For this review, take the finished solid that the model builds, in its own axes (mm). Face numbers are marked on the shaded views. Round coordinates to 2 decimals unless told otherwise and drop trailing zeros. Order: outer loops, then holes, each group sorted by start corner. A loop starts at its lowest first (then second) coordinate and runs counter-clockwise, first axis right, second up. Notation, with made-up numbers: M -23.5,43 L 18.5,43 A17 cw 18.5,75 Z; hole C 67,85.5 d8. An arc over 180 degrees is marked long. Put each result on its own line as item: value.
from build123d import *
from build123d.topology import SkipClean

# Parameters (mm, degrees)
SKETCH1_W               = 50
SKETCH1_H               = 50
SKETCH1_R               = 16.3
SKETCH1_R_2             = 2.35
BOSS_EXTRUDE1_DEPTH     = 53.6
CUT_EXTRUDE1_DEPTH      = 66.015075175
CUT_EXTRUDE1_DEPTH_BACK = 66.015075175
SKETCH2_R               = 31.75
BOSS_EXTRUDE3_START     = 60
BOSS_EXTRUDE3_DEPTH     = 60
SKETCH12_W              = 60
SKETCH12_H              = 66
CUT_EXTRUDE7_DEPTH      = 8
CUT_EXTRUDE5_DEPTH      = 107.409398132
CUT_EXTRUDE5_DEPTH_BACK = 107.409398132
SKETCH9_R               = 2.25
CUT_EXTRUDE6_DEPTH      = 97.358246028
CUT_EXTRUDE6_DEPTH_BACK = 10
SKETCH10_R              = 2.8
FILLET1_R               = 8


with BuildPart() as part:
    # Sketch1 → Boss-Extrude1 (new body)
    with BuildSketch(Plane.XY):
        with Locations((0, -2)):
            Rectangle(SKETCH1_W, SKETCH1_H)
        with Locations((0, -2)):
            Circle(SKETCH1_R, mode=Mode.SUBTRACT)
        with Locations((-20, 18)):
            Circle(SKETCH1_R_2, mode=Mode.SUBTRACT)
        with Locations((20, 18)):
            Circle(SKETCH1_R_2, mode=Mode.SUBTRACT)
        with Locations((20, -22)):
            Circle(SKETCH1_R_2, mode=Mode.SUBTRACT)
        with Locations((-20, -22)):
            Circle(SKETCH1_R_2, mode=Mode.SUBTRACT)
    extrude(amount=BOSS_EXTRUDE1_DEPTH)

    # Sketch2 → Cut-Extrude1 (cut, two sides: drawn at the far end of the back side and taken through both)
    with BuildSketch(Plane(origin=(0, 0, 0), x_dir=(0, 0, -1), z_dir=(1, 0, 0)).offset(-CUT_EXTRUDE1_DEPTH_BACK)):
        Circle(SKETCH2_R)
    extrude(amount=CUT_EXTRUDE1_DEPTH + CUT_EXTRUDE1_DEPTH_BACK, mode=Mode.SUBTRACT)

    # Sketch4 → Boss-Extrude3 (add)
    with SkipClean():  # the faces are left unmerged after this step: merging them gives an invalid solid
        with BuildSketch(Plane(origin=(25, 0, 0), x_dir=(0, 0, -1), z_dir=(1, 0, 0)).offset(BOSS_EXTRUDE3_START)):
            with BuildLine():
                Line((-53.6, -27), (-53.6, -35))
                Line((-53.6, -35), (-16.705163872, -35))
                Line((-16.705163872, -35), (-16.705163872, -27))
                ThreePointArc((-16.705163872, -27), (-31.580822619, -3.273246506), (-21.887496431, 23))
                Line((-21.887496431, 23), (-21.887496431, 31))
                Line((-21.887496431, 31), (-53.6, 31))
                Line((-53.6, 31), (-53.6, 23))
                Line((-53.6, 23), (-53.6, -27))
            make_face()
        extrude(amount=-BOSS_EXTRUDE3_DEPTH)

    # Sketch12 → Cut-Extrude7 (cut)
    with SkipClean():  # the faces are left unmerged after this step: merging them gives an invalid solid
        with BuildSketch(Plane.XY.offset(53.6)):
            with Locations((55, -2)):
                Rectangle(SKETCH12_W, SKETCH12_H)
        extrude(amount=-CUT_EXTRUDE7_DEPTH, mode=Mode.SUBTRACT)

    # Sketch9 → Cut-Extrude5 (cut, two sides: drawn at the far end of the back side and taken through both)
    with SkipClean():  # the faces are left unmerged after this step: merging them gives an invalid solid
        with BuildSketch(Plane.XY.offset(-CUT_EXTRUDE5_DEPTH_BACK)):
            with Locations(Location((30, 22, 0), (0, 0, 153.612200039))):
                Circle(SKETCH9_R)
            with Locations(Location((70, 22, 0), (0, 0, 153.612200039))):
                Circle(SKETCH9_R)
            with Locations(Location((70, -18, 0), (0, 0, 180))):
                Circle(SKETCH9_R)
            with Locations(Location((30, -18, 0), (0, 0, 180))):
                Circle(SKETCH9_R)
        extrude(amount=CUT_EXTRUDE5_DEPTH + CUT_EXTRUDE5_DEPTH_BACK, mode=Mode.SUBTRACT)

    # Sketch10 → Cut-Extrude6 (cut, two sides: drawn at the far end of the back side and taken through both)
    with SkipClean():  # the faces are left unmerged after this step: merging them gives an invalid solid
        with BuildSketch(Plane.XY.offset(45.6).offset(-CUT_EXTRUDE6_DEPTH_BACK)):
            with Locations((50, 4.5)):
                Circle(SKETCH10_R)
            with Locations((50, -8.5)):
                Circle(SKETCH10_R)
        extrude(amount=CUT_EXTRUDE6_DEPTH + CUT_EXTRUDE6_DEPTH_BACK, mode=Mode.SUBTRACT)

    # Fillet1
    # the kernel refuses this fillet: 8 mm, written as the material it adds along each edge
    with BuildSketch(Plane(origin=(25, 23, 21.887496431), x_dir=(-1, 0, 0), z_dir=(0, 0, 1))) as fillet1_piece_1:
        with BuildLine():
            CenterArc((FILLET1_R, -FILLET1_R), FILLET1_R, 90, 90)
            Line((0, -FILLET1_R), (0, 0))
            Line((0, 0), (FILLET1_R, 0))
        make_face()
    extrude(amount=23.712503569)
    with BuildSketch(Plane(origin=(25, -27, 16.705163872), x_dir=(-1, 0, 0), z_dir=(0, 0, 1))) as fillet1_piece_2:
        with BuildLine():
            CenterArc((FILLET1_R, FILLET1_R), FILLET1_R, 180, 90)
            Line((0, FILLET1_R), (0, 0))
            Line((0, 0), (FILLET1_R, 0))
        make_face()
    extrude(amount=28.894836128)


solid = part.part
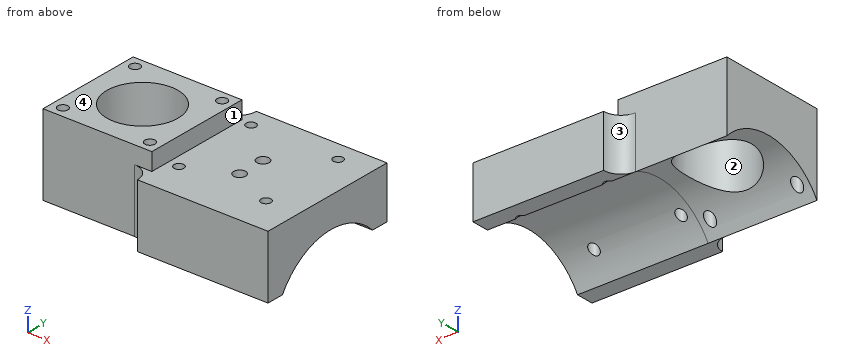
(1) Insertion check: pin 1 Ø7.5 at (x, y) = (20, 18) entering from -Z; pin 2 Ø4 at (x, y) = (27, -18) entering from -Z; pin 3 Ø1 at (x, z) = (46.5, 48) entering from +Y; pin 4 Ø6 at (x, y) = (30, -18) entering from +Z. Each pin has a flat end and moves straight along its axis. Give the tip position at first contact, or say it passes through.
A:
pin 1: stops at z = 23.13
pin 2: stops at z = 24.66
pin 3: passes through
pin 4: stops at z = 45.6
(2) To check wall thickness, follow L1, parallel to X at y = 22, z = 33; L2, parallel to Y at x = 30, z = 38; L3, parallel to Y at x = 20, z = 47. State the ranges of each line that lie inside material, in increasing order.
A:
L1: x = -25 to 27.75, 32.25 to 67.75, 72.25 to 85
L2: y = -35 to -20.25, -15.75 to 19.75, 24.25 to 31
L3: y = -27 to -24.35, -19.65 to 15.65, 20.35 to 23
(3) Add section A-A on y = 4.5. Give the boundary of the cut face in (x, z).
A:
outline: M -25,31.43 L -14.95,31.43 L -14.95,53.6 L -25,53.6 Z; M 14.95,31.43 L 85,31.43 L 85,45.6 L 52.8,45.6 L 52.8,35.6 L 47.2,35.6 L 47.2,45.6 L 25,45.6 L 25,53.6 L 14.95,53.6 Z
(4) Add section B-B on x = 0. Give the boundary of the cut face in (y, z).
A:
outline: M -27,16.71 A31.75 cw -18.3,25.95 L -18.3,53.6 L -27,53.6 Z; M 14.3,28.35 A31.75 cw 23,21.89 L 23,53.6 L 14.3,53.6 Z
(5) Draft analysis for pull direction X (two halves, no side actions). For the marked faces 1, 2, 3 and 4, state which applies: released by +X, released by -X, zero draft, split by the parting line, or undercut.
A:
face 1: released by +X
face 2: undercut
face 3: released by -X
face 4: zero draft
(6) Add section D-D on x = 70. Give the boundary of the cut face in (y, z), then the cut area to 3 significant figures.
A:
outline: M -35,16.71 L -27,16.71 A31.75 cw -20.25,24.45 L -20.25,45.6 L -35,45.6 Z; M -15.75,27.57 A31.75 cw 19.75,24.86 L 19.75,45.6 L -15.75,45.6 Z; M 24.25,21.89 L 31,21.89 L 31,45.6 L 24.25,45.6 Z
area: 1,110 mm2
(7) Add section C-C on z = 48. Give the boundary of the cut face in (x, y), then the cut area to 3 significant figures.
A:
outline: M -25,-27 L 25,-27 L 25,23 L -25,23 Z; hole C -20,-22 d4.7; hole C -20,18 d4.7; hole C 0,-2 d32.6; hole C 20,-22 d4.7; hole C 20,18 d4.7
area: 1,600 mm2
